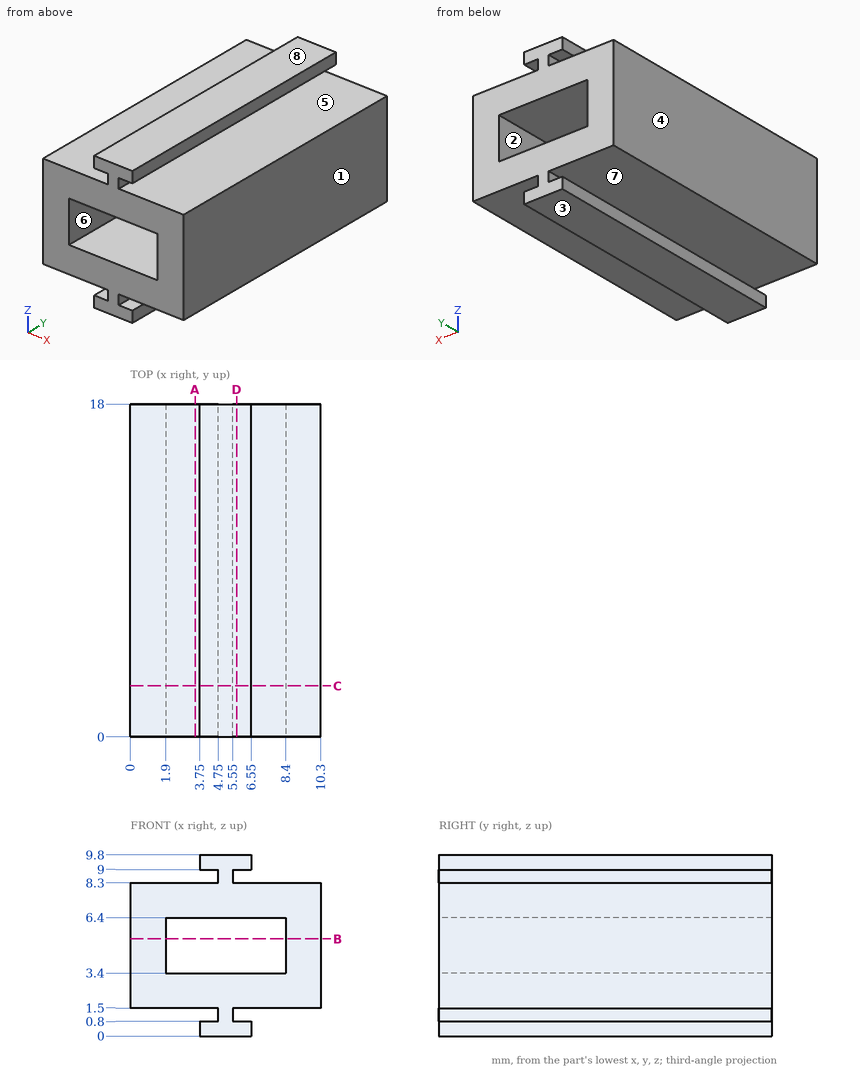
Verification items for this drawing (mm, ordinates from the low corner). A direction names the side the tool comes from. Round coordinates to 2 decimals unless told otherwise and drop trailing zeros. Loops run counter-clockwise (first coordinate to the right, second up) from the corner with the lowest first, then second, coordinate; pieces in that order, holes last. Notation, with made-up numbers: (-8, 48.25) -> (40, 48.25) arc R16 cw to (40, 71.25) -> close; hole circle Ø3 at (17.5, -2). An arc over 180 degrees is marked (long way). Answer in a Markdown table with one row per item.
Q1. Go/stop test with flat-tipped pins: P1, Ø0.9, axis at y = 12.5, z = 9.5, coming from the +X side; P2, Ø1.4, axis at x = 9, y = 8.5, coming from the +Z side; P3, Ø0.9, axis at y = 6.5, z = 0.5, coming from the -X side. Record where each tip stops, or that it passes through.
Data:
| item | result |
|---|---|
| P1 | stops at x = 6.55 |
| P2 | stops at z = 8.3 |
| P3 | stops at x = 3.75 |
Q2. Release check for a two-part mould opening along Z. For the marked faces 1, 2 and 3 record: released by +Z, released by -Z, zero draft, split by the parting line, or undercut.
Data:
| item | result |
|---|---|
| face 1 | zero draft |
| face 2 | undercut |
| face 3 | released by -Z |
Q3. Sectioned sample at A-A on x = 3.5. Enter the section's corners in (y, z).
Data:
| item | result |
|---|---|
| outline | (0, 1.5) -> (18, 1.5) -> (18, 3.4) -> (0, 3.4) -> close; (0, 6.4) -> (18, 6.4) -> (18, 8.3) -> (0, 8.3) -> close |
Q4. Set-up check for the marked faces 4, 5, 6, 7 and 8: record each of +Z, -Z, +X, -X, +Y, -Y from which the full face is reachable in a straight line by a thin tool's end or side.
Data:
| item | result |
|---|---|
| face 4 | +Z, -Z, -X, +Y, -Y |
| face 5 | +X, +Y, -Y |
| face 6 | +Y, -Y |
| face 7 | -X, +Y, -Y |
| face 8 | +Z, +X, -X, +Y, -Y |
Q5. Sectioned sample at C-C on y = 2.75. Enter the section's corners in (x, z), then the cut area to 3 significant figures.
Data:
| item | result |
|---|---|
| outline | (0, 1.5) -> (4.75, 1.5) -> (4.75, 0.8) -> (3.75, 0.8) -> (3.75, 0) -> (6.55, 0) -> (6.55, 0.8) -> (5.55, 0.8) -> (5.55, 1.5) -> (10.3, 1.5) -> (10.3, 8.3) -> (5.55, 8.3) -> (5.55, 9) -> (6.55, 9) -> (6.55, 9.8) -> (3.75, 9.8) -> (3.75, 9) -> (4.75, 9) -> (4.75, 8.3) -> (0, 8.3) -> close; hole (1.9, 3.4) -> (8.4, 3.4) -> (8.4, 6.4) -> (1.9, 6.4) -> close |
| area | 56.1 mm^2 |
Q6. Sectioned sample at B-B on z = 5.25. Enter the section's corners in (x, y).
Data:
| item | result |
|---|---|
| outline | (0, 0) -> (1.9, 0) -> (1.9, 18) -> (0, 18) -> close; (8.4, 0) -> (10.3, 0) -> (10.3, 18) -> (8.4, 18) -> close |
Q7. Sectioned sample at D-D on x = 5.75. Enter the section's corners in (y, z), then the cut area to 3 significant figures.
Data:
| item | result |
|---|---|
| outline | (0, 0) -> (18, 0) -> (18, 0.8) -> (0, 0.8) -> close; (0, 1.5) -> (18, 1.5) -> (18, 3.4) -> (0, 3.4) -> close; (0, 6.4) -> (18, 6.4) -> (18, 8.3) -> (0, 8.3) -> close; (0, 9) -> (18, 9) -> (18, 9.8) -> (0, 9.8) -> close |
| area | 97.2 mm^2 |
Q8. Thickness scan on L1, parallel to X at y = 15.25, z = 5.25; L2, parallel to Z at x = 8.25, y = 13; L3, parallel to Z at x = 5.5, y = 16.5. Record the ranges inside material, lowest first.
Data:
| item | result |
|---|---|
| L1 | x = 0 to 1.9, 8.4 to 10.3 |
| L2 | z = 1.5 to 3.4, 6.4 to 8.3 |
| L3 | z = 0 to 3.4, 6.4 to 9.8 |
